from build123d import *

# Parameters (mm, degrees)
SKETCH_1_W           = 224
SKETCH_1_H           = 63
EXTRUDE_6_DEPTH      = 3
SKETCH_1_3_W         = 230
SKETCH_1_3_H         = 69
SKETCH_1_3_W_2       = 224
SKETCH_1_3_H_2       = 63
EXTRUDE_1_DEPTH      = 76
SKETCH_6_W           = 23.5
SKETCH_6_H           = 35
SKETCH_6_W_2         = 24
CUT_EXTRUDE_1_DEPTH  = 4
SKETCH_8_W           = 14
SKETCH_8_H           = 14
EXTRUDE_8_DEPTH      = 40
SKETCH_11_R          = 2
CUT_EXTRUDE_2_DEPTH  = 10
CUT_EXTRUDE_4_DEPTH  = 3
SKETCH_14_W          = 14
SKETCH_14_H          = 14
EXTRUDE_9_DEPTH      = 44.5
SKETCH_15_R          = 2
CUT_EXTRUDE_5_DEPTH  = 13
CUT_EXTRUDE_11_DEPTH = 6
EXTRUDE_10_DEPTH     = 5
EXTRUDE_11_DEPTH     = 5
SKETCH_30_W          = 230
SKETCH_30_H          = 2
EXTRUDE_13_DEPTH     = 76
FILLET_3_R           = 2
SKETCH_31_R          = 2.75
CUT_EXTRUDE_13_DEPTH = 2.5
SKETCH_28_R          = 1.75
CUT_EXTRUDE_14_DEPTH = 2.5
CUT_EXTRUDE_3_DEPTH  = 3


with BuildPart() as part:
    # Sketch 1 → Extrude 6 (new body)
    with BuildSketch(Plane.XY):
        Rectangle(SKETCH_1_W, SKETCH_1_H)
    extrude(amount=EXTRUDE_6_DEPTH)

    # Sketch 1_3 → Extrude 1 (add)
    with BuildSketch(Plane.XY):
        Rectangle(SKETCH_1_3_W, SKETCH_1_3_H)
        Rectangle(SKETCH_1_3_W_2, SKETCH_1_3_H_2, mode=Mode.SUBTRACT)
    extrude(amount=EXTRUDE_1_DEPTH)

    # Sketch 6 → Cut-Extrude 1 (cut)
    with BuildSketch(Plane(origin=(0, 0, 0), x_dir=(-1, 0, 0), z_dir=(0, 0, -1))):
        with Locations((-83.8, -6)):
            Rectangle(SKETCH_6_W, SKETCH_6_H)
        with Locations((-55.55, -7)):
            Rectangle(SKETCH_6_W_2, SKETCH_6_H)
        with Locations((-14.25, -7)):
            Rectangle(SKETCH_6_W_2, SKETCH_6_H)
        with Locations((14.25, -7)):
            Rectangle(SKETCH_6_W_2, SKETCH_6_H)
        with Locations((55.55, -7)):
            Rectangle(SKETCH_6_W_2, SKETCH_6_H)
        with Locations((83.8, -7)):
            Rectangle(SKETCH_6_W, SKETCH_6_H)
    extrude(amount=-CUT_EXTRUDE_1_DEPTH, mode=Mode.SUBTRACT)

    # Sketch 8 → Extrude 8 (add)
    with BuildSketch(Plane.XY.offset(3)):
        with Locations((-105, 24.5)):
            Rectangle(SKETCH_8_W, SKETCH_8_H)
        with Locations((-105, -24.5)):
            Rectangle(SKETCH_8_W, SKETCH_8_H)
    extrude(amount=EXTRUDE_8_DEPTH)

    # Sketch 11 → Cut-Extrude 2 (cut)
    with BuildSketch(Plane.XY.offset(43)):
        with Locations((-105.25, 24.51)):
            Circle(SKETCH_11_R)
        with Locations((-105.25, -24.51)):
            Circle(SKETCH_11_R)
    extrude(amount=-CUT_EXTRUDE_2_DEPTH, mode=Mode.SUBTRACT)

    # Sketch 12_2 → Cut-Extrude 4 (cut)
    with BuildSketch(Plane.XY.offset(43)):
        Polygon((-107.270725942, 28.01), (-109.291451884, 24.51), (-107.270725942, 21.01), (-103.229274058, 21.01), (-101.208548116, 24.51), (-103.229274058, 28.01), align=None)
        Polygon((-101.208548116, -24.51), (-103.229274058, -21.01), (-107.270725942, -21.01), (-109.291451884, -24.51), (-107.270725942, -28.01), (-103.229274058, -28.01), align=None)
    extrude(amount=-CUT_EXTRUDE_4_DEPTH, mode=Mode.SUBTRACT)

    # Sketch 14 → Extrude 9 (add)
    with BuildSketch(Plane(origin=(0, 0, 0), x_dir=(-1, 0, 0), z_dir=(0, 0, -1))):
        with Locations((-105, 24.5)):
            Rectangle(SKETCH_14_W, SKETCH_14_H)
        with Locations((-105, -24.5)):
            Rectangle(SKETCH_14_W, SKETCH_14_H)
    extrude(amount=-EXTRUDE_9_DEPTH)

    # Sketch 15 → Cut-Extrude 5 (cut)
    with BuildSketch(Plane.XY.offset(44.5)):
        with Locations((105.25, 24.514472103)):
            Circle(SKETCH_15_R)
        with Locations((105.25, -24.51)):
            Circle(SKETCH_15_R)
    extrude(amount=-CUT_EXTRUDE_5_DEPTH, mode=Mode.SUBTRACT)

    # Sketch 16 → Cut-Extrude 11 (cut)
    with BuildSketch(Plane.XY.offset(44.5)):
        Polygon((103.229274058, 21.014472103), (107.270725942, 21.014472103), (109.291451884, 24.514472103), (107.270725942, 28.014472103), (103.229274058, 28.014472103), (101.208548116, 24.514472103), align=None)
        Polygon((103.229274058, -28.01), (107.270725942, -28.01), (109.291451884, -24.51), (107.270725942, -21.01), (103.229274058, -21.01), (101.208548116, -24.51), align=None)
    extrude(amount=-CUT_EXTRUDE_11_DEPTH, mode=Mode.SUBTRACT)

    # Sketch 21 → Extrude 10 (add, symmetric)
    with BuildSketch(Plane.ZY.offset(34.5)):
        Polygon((3, 31.5), (33, 31.5), (3, 16.5), align=None)
        Polygon((3, -16.5), (3, -31.5), (33, -31.5), align=None)
    extrude(amount=EXTRUDE_10_DEPTH, both=True)

    # Sketch 22 → Extrude 11 (add, symmetric)
    with BuildSketch(Plane(origin=(34.5, 0, 0), x_dir=(0, 0, -1), z_dir=(1, 0, 0))):
        Polygon((-3, 31.5), (-3, 16.5), (-33, 31.5), align=None)
        Polygon((0, -16.5), (0, -31.5), (-30, -31.5), align=None)
    extrude(amount=EXTRUDE_11_DEPTH, both=True)

    # Sketch 30 → Extrude 13 (add)
    with BuildSketch(Plane(origin=(0, 0, 0), x_dir=(-1, 0, 0), z_dir=(0, 0, -1))):
        with Locations((0, -35.5)):
            Rectangle(SKETCH_30_W, SKETCH_30_H)
    extrude(amount=-EXTRUDE_13_DEPTH)

    # Fillet 3
    fillet_3_edges = [part.edges().sort_by_distance(p)[0] for p in [
        (0, 34.5, 0),
        (0, -36.5, 0),
    ]]
    fillet(fillet_3_edges, radius=FILLET_3_R)

    # Sketch 31 → Cut-Extrude 13 (cut)
    with BuildSketch(Plane.XZ.offset(36.5)):
        with Locations(Location((-85.5, 68, 0), (0, 0, 270))):
            Circle(SKETCH_31_R)
        with Locations(Location((85.5, 68, 0), (0, 0, 270))):
            Circle(SKETCH_31_R)
    extrude(amount=-CUT_EXTRUDE_13_DEPTH, mode=Mode.SUBTRACT)

    # Sketch 28 → Cut-Extrude 14 (cut)
    with BuildSketch(Plane(origin=(0, -31.5, 0), x_dir=(1, 0, 0), z_dir=(0, 1, 0))):
        with Locations(Location((85.5, -68, 0), (0, 0, 270))):
            Circle(SKETCH_28_R)
        with Locations(Location((-85.5, -68, 0), (0, 0, 270))):
            Circle(SKETCH_28_R)
    extrude(amount=-CUT_EXTRUDE_14_DEPTH, mode=Mode.SUBTRACT)

    # Sketch 12 → Cut-Extrude 3 (cut)
    with BuildSketch(Plane.XY.offset(43)):
        Polygon((-107.270725942, 28.01), (-109.291451884, 24.51), (-107.270725942, 21.01), (-103.229274058, 21.01), (-101.208548116, 24.51), (-103.229274058, 28.01), align=None)
        Polygon((-101.208548116, -24.51), (-103.229274058, -21.01), (-107.270725942, -21.01), (-109.291451884, -24.51), (-107.270725942, -28.01), (-103.229274058, -28.01), align=None)
    extrude(amount=-CUT_EXTRUDE_3_DEPTH, mode=Mode.SUBTRACT)


solid = part.part
Here's how the part is built. I have some questions about the finished solid (model axes, mm). A direction names the side the tool comes from. Round coordinates to 2 decimals unless told otherwise and drop trailing zeros. Loops run counter-clockwise (first coordinate to the right, second up) from the corner with the lowest first, then second, coordinate; pieces in that order, holes last.
1. If I drill on line 1 along Y through (x, z) = (-105.25, 37.5); line 2 along X through (y, z) = (-33.2, 68); line 3 along X through (y, z) = (11.5, 59), over which ranges is the centre line in solid material (lowest first)?
Answer list:
line 1: y = -36.5 to -26.51, -22.51 to -17.5, 17.5 to 22.51, 26.51 to 34.5
line 2: x = -115 to -87.25, -83.75 to 83.75, 87.25 to 115
line 3: x = -115 to -112, 112 to 115
2. We'd pull the mould along X, two halves only. Please class faces 1 (the face through (2, -36.5, 38)), 2 (the face through (-115, -1, 37)), 3 (the face through (-29.5, 27, 12)): +X half, -X half, draft (parallel to the pull), parting line (faces both ways), or undercut.
Answer list:
face 1: draft
face 2: -X half
face 3: undercut
3. If we section it at C-C on z = 50: Write out the boundary of the cut face in (x, y).
Answer list:
outline: (-115, -36.5) - (115, -36.5) - (115, 34.5) - (-115, 34.5) - close; hole (-112, -31.5) - (112, -31.5) - (112, 31.5) - (-112, 31.5) - close
4. If we section it at A-A on x = 50: Write out the boundary of the cut face in (y, z).
Answer list:
outline: (-36.5, 2) arc R2 ccw to (-34.5, 0) - (-24.5, 0) - (-24.5, 3) - (-31.5, 3) - (-31.5, 76) - (-36.5, 76) - close; (10.5, 0) - (32.5, 0) arc R2 ccw to (34.5, 2) - (34.5, 76) - (31.5, 76) - (31.5, 3) - (10.5, 3) - close
5. For P1, Ø5.5, axis at x = -105, y = -24, coming from the +Z side, with a flat end and sliding along its axis, tell me the tip position at first contact or that it passes through.
Answer list:
P1: stops at z = 40
6. If we section it at B-B on y = -14: Count the separate pieces of the cut face and the enclosed holes in it, plus the area to 3 significant figures.
Answer list:
separate pieces: 7
enclosed holes: 0
area: 699 mm2
7. Which directions (+Z, -Z, +X, -X, +Y, -Y) give clear straight access to the entire face, cutting with the end or side of a thin tool? Please do faces 4 (the face through (-2, 34.5, 38)), 5 (the face through (107.158, 25.115, 35.049)).
Answer list:
face 4: +Z, -Z, +X, -X, +Y
face 5: +Z
